Geometry: final body of the model. Coordinates: model frame, mm. A direction names the side the tool comes from. Give positions to 0.01 mm unless a question says otherwise; leave off trailing zeros. Loops run counter-clockwise (first coordinate to the right, second up) from the corner with the lowest first, then second, coordinate; pieces in that order, holes last.
from build123d import *

# Parameters (mm, degrees)
BOSS_EXTRUDE1_DEPTH = 5


with BuildPart() as part:
    # Sketch1 → Boss-Extrude1 (new body)
    with BuildSketch(Plane(origin=(0, 0, 0), x_dir=(1, 0, 0), z_dir=(0, 1, 0))):
        Polygon((-339.799413006, 126.304683991), (-339.799413006, 191.992892094), (-303.040106148, 191.992892094), (-290.400599698, 179.353385644), (-308.734522065, 161.019463277), (-294.552751732, 146.837692944), (-294.552751732, 136.018956443), (-301.910980799, 136.018956443), (-301.910980799, 147.500427473), (-313.95979318, 159.549239854), (-327.618746258, 159.549239854), (-320.592033082, 166.575953029), (-311.753745416, 166.575953029), (-301.268571849, 177.061126596), (-308.734454598, 184.527009345), (-329.704801732, 184.527009345), (-329.704801732, 142.586315078), align=None)
    extrude(amount=BOSS_EXTRUDE1_DEPTH)


solid = part.part
Item 1: Section query B-B on x = -317. Return loops of the section in (y, z).
Values follow:
outline: (0, -191.99) - (5, -191.99) - (5, -184.53) - (0, -184.53) - close; (0, -166.58) - (5, -166.58) - (5, -159.55) - (0, -159.55) - close
Item 2: Pin query (flat end, axial travel): pin 1 (1.5 mm diameter, centred on x = -298, y = 1.5, fed in from +Z); pin 2 (2.5 mm diameter, centred on x = -318, y = 3.5, fed in from +Z); pin 3 (3 mm diameter, centred on y = 4, z = -154, fed in from +X). Return the tip coordinate at first contact, or that it passes through.
Values follow:
pin 1: stops at z = -136.02
pin 2: stops at z = -159.55
pin 3: stops at x = -300.22
Item 3: Set-up query: faces 5 (the face through (-304.95, 2.46, -180.74)), 6 (the face through (-329.705, 2, -164)), 7 (the face through (-298, 2, -136.019)). Return all of +Z, -Z, +X, -X, +Y, -Y with unobstructed straight access to the full face (end or side cutting, diameter ignored); none if empty.
Values follow:
face 5: +Y, -Y
face 6: +Z, +Y, -Y
face 7: +Z, +X, +Y, -Y
Item 4: Ray query, probe 1 along Z at (x, y) = (-316, 4.7); probe 2 along Z at (x, y) = (-308, 2.7); probe 3 along Z at (x, y) = (-302.5, 2.3). Return the intervals inside material, ascending.
Values follow:
probe 1: z = -191.99 to -184.53, -166.58 to -159.55
probe 2: z = -191.99 to -183.79, -170.33 to -161.75, -160.28 to -153.59
probe 3: z = -191.45 to -178.29, -175.83 to -167.25, -154.78 to -148.09
Item 5: Draft query along Z for faces 1 (the face through (-316, 2, -166.576)), 2 (the face through (-299.439, 2.465, -170.315)), 3 (the face through (-334.68, 2.46, -134.56)), 4 (the face through (-320, 5, -160)). Return one class per face: +Z half, -Z half, draft (parallel to the pull), parting line (faces both ways), or undercut.
Values follow:
face 1: undercut
face 2: undercut
face 3: +Z half
face 4: draft
Item 6: Section query D-D on x = -305.5. Return loops of the section in (y, z).
Values follow:
outline: (0, -191.99) - (5, -191.99) - (5, -181.29) - (0, -181.29) - close; (0, -172.83) - (5, -172.83) - (5, -164.25) - (0, -164.25) - close; (0, -157.78) - (5, -157.78) - (5, -151.09) - (0, -151.09) - close
Item 7: Section query C-C on y = 3.6. Return loops of the section in (x, z), plus the area to 3 significant figures.
Values follow:
outline: (-339.8, -191.99) - (-303.04, -191.99) - (-290.4, -179.35) - (-308.73, -161.02) - (-294.55, -146.84) - (-294.55, -136.02) - (-301.91, -136.02) - (-301.91, -147.5) - (-313.96, -159.55) - (-327.62, -159.55) - (-320.59, -166.58) - (-311.75, -166.58) - (-301.27, -177.06) - (-308.73, -184.53) - (-329.7, -184.53) - (-329.7, -142.59) - (-339.8, -126.3) - close
area: 1,280 mm2
Item 8: Section query A-A on z = -146. Return loops of the section in (x, y).
Values follow:
outline: (-339.8, 0) - (-329.7, 0) - (-329.7, 5) - (-339.8, 5) - close; (-301.91, 0) - (-294.55, 0) - (-294.55, 5) - (-301.91, 5) - close
